Can you work these out from the model? Positions are in its coordinate system, mm. A direction names the side the tool comes from. Give positions to 0.01 mm unless a question says otherwise; leave off trailing zeros. Loops run counter-clockwise (first coordinate to the right, second up) from the corner with the lowest first, then second, coordinate; pieces in that order, holes last. Notation, with made-up numbers: (-30.5, 84) - (8.5, 84) arc R19 ccw to (8.5, 88) - close; hole circle Ø1 at (22.5, -29). An arc over 180 degrees is marked (long way). Answer as a JSON object with one key per item and string values.
Autodesk Inventor part; units mm, degrees
ref_plane "YZ Plane" through (0, 0, 0) normal (1, 0, 0) x (0, 1, 0)
ref_plane "XZ Plane" through (0, 0, 0) normal (0, 1, 0) x (-1, 0, 0)
ref_plane "XY Plane" through (0, 0, 0) normal (0, 0, 1) x (1, 0, 0)
sketch "Sketch1" plane through (0, 0, 0) normal (1, 0, 0) x (0, 1, 0)
  line L0 (0, 0) -> (4, 0)
  line L1 (0, 0) -> (0, -11)
  line L2 (0, -11) -> (4, -11)
  line L3 (4, -11) -> (4, -7.5)
  line L4 (2, -4) -> (4, 0)
  line L5 (4, -7.5) -> (2, -4)
  line L6 (4, -7.5) -> (4, -7.5)
  dimension "d1" = 11
  dimension "d2" = 4
  dimension "d3" = 3.5
  dimension "d11" = 4
  dimension "d12" = 2
  dimension "d13" = 4
  dimension "d14" = 0
  dimension "d15" = 3.5
revolve "Revolution1" add sketch "Sketch1" angle 360 about axis through (0, 0, 0) along (0, 0, -1)
sketch "Sketch2" plane through (0, 0, -11) normal (0, 0, -1) x (-1, 0, 0)
  arc A0 (1.362, -0.975) -> (-1.362, -0.975) centre (0, 0) ccw
  line L0 (-1.9022, -0.975) -> (1.9927, -0.975)
  dimension "d7" = 3.35
  dimension "d8" = 2.65
extrude "Extrusion1" cut sketch "Sketch2" against normal blind 9.5
sketch "Sketch3" plane through (0, 0, 0) normal (0, 0, 1) x (1, 0, 0)
  circle A0 centre (0, 0) radius 4
  point P0 (0, 0)
extrude "Extrusion2" cut sketch "Sketch3" against normal blind 1
chamfer "Chamfer1" distance 0.5 angle 45 1 edges at (0, -3.5, -1)
properties part number "drive-pulley"
1) Imagine slicing it at A-A on y = 0. Write out the boundary of the cut face in (x, z).
Check sheet entries:
{"outline": "(-4, -11) - (-1.68, -11) - (-1.68, -1.5) - (1.68, -1.5) - (1.68, -11) - (4, -11) - (4, -7.5) - (2, -4) - (3.28, -1.45) - (3, -1) - (-3, -1) - (-3.28, -1.45) - (-2, -4) - (-4, -7.5) - close"}
2) I'm going to push flat-ended pins straight in: P1, Ø3, axis at x = 3, z = -8, coming from the -Y side; P2, Ø1.5, axis at y = -1.5, z = -4, coming from the -X side; P3, Ø1.3, axis at x = 0, y = 0.5, coming from the -Z side. Where does each tip first touch, or does it pass through?
Check sheet entries:
{"P1": "y = -3.71", "P2": "x = -2.09", "P3": "z = -1.5"}
3) I need wall thicknesses on L1, parallel to X at y = 0, z = -8.5; L2, parallel to Y at x = 0, z = -5.75 (3 decimals); L3, parallel to Z at x = 0.5, y = -0.5. Which ranges of each line are inside material? Lowest first, please.
Check sheet entries:
{"L1": "-4 to -1.68, 1.68 to 4", "L2": "-3 to -0.975, 1.675 to 3", "L3": "-1.5 to -1"}
4) Which directions (+Z, -Z, +X, -X, +Y, -Y) give clear straight access to the entire face, cutting with the end or side of a thin tool? Please do faces 5 (the flat face through (0, 0, -1.5)), 6 (the cylindrical face through (3.905, -0.867, -9.226)), 7 (the conical face through (-2.062, -0.271, -3.84)).
Check sheet entries:
{"face 5": "-Z", "face 6": "+Z, -Z", "face 7": "none"}
5) Imagine slicing it at D-D on z = -4.5. Write out the boundary of the cut face in (x, y) (3 decimals).
Check sheet entries:
{"outline": "circle Ø4.571 at (0, 0); hole (-1.362, -0.975) - (1.362, -0.975) arc R1.675 ccw (long way) to start"}
6) If we mould it in two halves opening along X, with no side actions, what happens to faces 1 (the flat face through (0, 0, -1)), 2 (the cylindrical face through (-0.051, 1.674, -6.316)), 3 (the conical face through (0.71, 2.24, -4.61)), 4 (the flat face through (0, -0.975, -6))? For each: released by +X, released by -X, zero draft, split by the parting line, or undercut.
Check sheet entries:
{"face 1": "zero draft", "face 2": "undercut", "face 3": "split by the parting line", "face 4": "undercut"}
7) Imagine slicing it at B-B on x = 0. Write out the boundary of the cut face in (y, z) (3 decimals).
Check sheet entries:
{"outline": "(-4, -11) - (-0.975, -11) - (-0.975, -1.5) - (1.675, -1.5) - (1.675, -11) - (4, -11) - (4, -7.5) - (2, -4) - (3.276, -1.447) - (3, -1) - (-3, -1) - (-3.276, -1.447) - (-2, -4) - (-4, -7.5) - close"}
8) Imagine slicing it at C-C on z = -10.5. Write out the boundary of the cut face in (x, y) (3 decimals).
Check sheet entries:
{"outline": "circle Ø8 at (0, 0); hole (-1.362, -0.975) - (1.362, -0.975) arc R1.675 ccw (long way) to start"}
